```python
from build123d import *

# Parameters (mm, degrees)
SKETCH1_R                 = 9.5
SKETCH1_R_2               = 2.1
BOSS_EXTRUDE1_DEPTH       = 9.26
BOSS_EXTRUDE2_OUTLINE_R   = 11.5
BOSS_EXTRUDE2_OUTLINE_R_2 = 2.1
BOSS_EXTRUDE2_DEPTH       = 20
SKETCH3_W                 = 6
SKETCH3_H                 = 2
CUT_EXTRUDE1_DEPTH        = 12
SKETCH4_R                 = 1.5
CUT_EXTRUDE2_DEPTH        = 39.953788006
SKETCH5_R                 = 1.5
CUT_EXTRUDE3_DEPTH        = 12


# Read off the part's stored shape, not the designer's step: Boss-Extrude2
with BuildPart() as part:
    # Sketch1 → Boss-Extrude1 (new body)
    with BuildSketch(Plane.XY):
        Circle(SKETCH1_R)
        Circle(SKETCH1_R_2, mode=Mode.SUBTRACT)
    extrude(amount=BOSS_EXTRUDE1_DEPTH)

    # Boss-Extrude2 outline → Boss-Extrude2 (add)
    with BuildSketch(Plane.XY.offset(9.26)):
        Circle(BOSS_EXTRUDE2_OUTLINE_R)
        Circle(BOSS_EXTRUDE2_OUTLINE_R_2, mode=Mode.SUBTRACT)
    extrude(amount=BOSS_EXTRUDE2_DEPTH)

    # Sketch3 → Cut-Extrude1 (cut)
    with BuildSketch(Plane.XY.offset(29.26)):
        with Locations((0, 5.422033923)):
            Rectangle(SKETCH3_W, SKETCH3_H)
        with Locations((0, -5.422033923)):
            Rectangle(SKETCH3_W, SKETCH3_H)
    extrude(amount=-CUT_EXTRUDE1_DEPTH, mode=Mode.SUBTRACT)

    # Sketch4 → Cut-Extrude2 (cut, through all)
    with BuildSketch(Plane(origin=(0, 11.5, 0), x_dir=(1, 0, 0), z_dir=(0, 1, 0))):
        with Locations(Location((0, -24.76, 0), (0, 0, 180))):
            Circle(SKETCH4_R)
    extrude(amount=-CUT_EXTRUDE2_DEPTH, mode=Mode.SUBTRACT)

    # Sketch5 → Cut-Extrude3 (cut)
    with BuildSketch(Plane(origin=(0, 0, 0), x_dir=(-1, 0, 0), z_dir=(0, 0, -1))):
        with Locations((0, 6)):
            Circle(SKETCH5_R)
        with Locations((5.196152423, -3)):
            Circle(SKETCH5_R)
        with Locations((-5.196152423, -3)):
            Circle(SKETCH5_R)
    extrude(amount=-CUT_EXTRUDE3_DEPTH, mode=Mode.SUBTRACT)


solid = part.part
```
Input: part model. Units: mm. Frame: model coordinates. A direction names the side the tool comes from. Coordinates: 2 decimals unless noted, no trailing zeros. Loops run counter-clockwise (first coordinate to the right, second up) from the corner with the lowest first, then second, coordinate; pieces in that order, holes last. Notation, with made-up numbers: M -27,45.5 L 28,45.5 A17 ccw 28,71.5 Z; hole C -35.5,77 d5. An arc over 180 degrees is marked long. Use a Markdown table: item, result. Add a question column.
1) Set-up query: faces 4 (the flat face through (-5, -3, 12)), 5 (the cylindrical face through (-0.806, 8.997, 26.025)), 6 (the flat face through (1, -6.422, 23)). Return all of +Z, -Z, +X, -X, +Y, -Y with unobstructed straight access to the full face (end or side cutting, diameter ignored); none if empty.
2) Pin query (flat end, axial travel): P1, Ø3, axis at x = -1, z = 23.5, coming from the +Y side; P2, Ø2, axis at y = 6, z = 24, coming from the -X side; P3, Ø2, axis at x = 9, z = 4.5, coming from the +Y side; P4, Ø0.6, axis at y = 5, z = 22, coming from the +X side. Return the tip coordinate at first contact, or that it passes through.
3) Section A-A, the plane z = 24.76. Return the cut outline in (x, y), plus the area to 3 significant figures.
4) Line query: L1, parallel to Y at x = -1.75, z = 21; L2, parallel to Z at x = 0, y = -3.5; L3, parallel to Z at x = -9.25, y = 4. Output: solid intervals per line, ascending. Write a range as from..to.
5) Section B-B, the plane y = -0.75. Return the cut outline in (x, z).
6) Section D-D, the plane x = 0. Give the number of separate pieces and of enclosed holes in the cut face, plus the area to 3 significant figures.
7) Draft query along Y for faces 1 (the cylindrical face through (-0.806, -2.925, 26.025)), 2 (the cylindrical face through (-1.5, 11.4, 19.1)), 3 (the flat face through (3, 5, 23)). Return one class per face: +Y half, -Y half, draft (parallel to the pull), parting line (faces both ways), or undercut.
8) Section C-C, the plane z = 21. Return the cut outline in (x, y).
Answer below:
| question | item | result |
|---|---|---|
| 1 | face 4 | -Z |
| 1 | face 5 | +Y, -Y |
| 1 | face 6 | +Z |
| 2 | P1 | y = 11.5 |
| 2 | P2 | x = -10.36 |
| 2 | P3 | y = 5.12 |
| 2 | P4 | x = 10.5 |
| 3 | outline | M -3,-6.42 L -3,-4.42 L -1.5,-4.42 L -1.5,-1.47 A2.1 cw -1.5,1.47 L -1.5,4.42 L -3,4.42 L -3,6.42 L -1.5,6.42 L -1.5,11.4 A11.5 ccw -1.5,-11.4 L -1.5,-6.42 Z; M 1.5,-11.4 A11.5 ccw 1.5,11.4 L 1.5,6.42 L 3,6.42 L 3,4.42 L 1.5,4.42 L 1.5,1.47 A2.1 cw 1.5,-1.47 L 1.5,-4.42 L 3,-4.42 L 3,-6.42 L 1.5,-6.42 Z |
| 3 | area | 332 mm2 |
| 4 | L1 | -11.37..-6.42, -4.42..-1.16, 1.16..4.42, 6.42..11.37 |
| 4 | L2 | 0..23.26, 26.26..29.26 |
| 4 | L3 | 9.26..29.26 |
| 5 | outline | M -11.48,9.26 L -9.47,9.26 L -9.47,0 L -1.96,0 L -1.96,29.26 L -11.48,29.26 Z; M 1.96,0 L 9.47,0 L 9.47,9.26 L 11.48,9.26 L 11.48,29.26 L 1.96,29.26 Z |
| 6 | separate pieces | 6 |
| 6 | enclosed holes | 0 |
| 6 | area | 385 mm2 |
| 7 | face 1 | draft |
| 7 | face 2 | parting line |
| 7 | face 3 | undercut |
| 8 | outline | C 0,0 d23; hole M -3,-6.42 L 3,-6.42 L 3,-4.42 L -3,-4.42 Z; hole M -3,4.42 L 3,4.42 L 3,6.42 L -3,6.42 Z; hole C 0,0 d4.2 |
